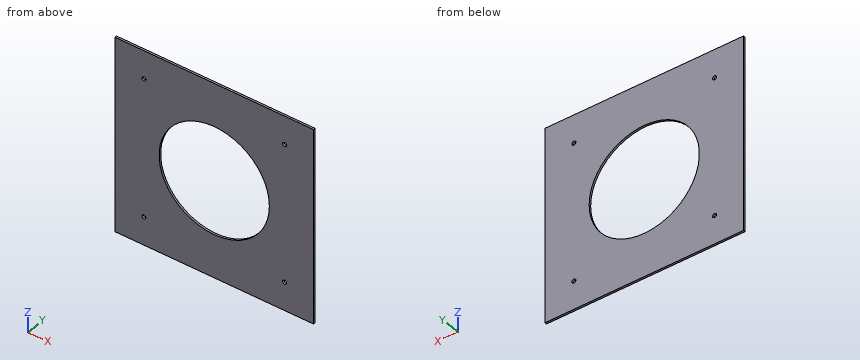
```python
from build123d import *

# Parameters (mm, degrees)
SKETCH1_W           = 98.782817332
SKETCH1_H           = 98.782817332
BOSS_EXTRUDE1_DEPTH = 1.000000032
SKETCH3_R           = 0.999998
CUT_EXTRUDE2_DEPTH  = 2.000000032
SKETCH8_R           = 27.432
CUT_EXTRUDE9_DEPTH  = 2.000000032


with BuildPart() as part:
    # Sketch1 → Boss-Extrude1 (new body)
    with BuildSketch(Plane(origin=(0, 0, 0), x_dir=(1, 0, 0), z_dir=(0, 1, 0))):
        Rectangle(SKETCH1_W, SKETCH1_H)
    extrude(amount=BOSS_EXTRUDE1_DEPTH)

    # Sketch3 → Cut-Extrude2 (cut, through all)
    with BuildSketch(Plane(origin=(0, 0, 0), x_dir=(1, 0, 0), z_dir=(0, 1, 0))):
        with Locations((35.001787507, 35.001787507)):
            Circle(SKETCH3_R)
        with Locations((35.001787507, -35.001787507)):
            Circle(SKETCH3_R)
        with Locations((-35.001787507, -35.001787507)):
            Circle(SKETCH3_R)
        with Locations((-35.001787507, 35.001787507)):
            Circle(SKETCH3_R)
    extrude(amount=CUT_EXTRUDE2_DEPTH, mode=Mode.SUBTRACT)

    # Sketch8 → Cut-Extrude9 (cut, through all)
    with BuildSketch(Plane(origin=(0, 0, 0), x_dir=(1, 0, 0), z_dir=(0, 1, 0))):
        Circle(SKETCH8_R)
    extrude(amount=CUT_EXTRUDE9_DEPTH, mode=Mode.SUBTRACT)


solid = part.part
```
Design review of the part built by this model. Coordinates are the model's own, in mm. Coordinates: 2 decimals unless noted, no trailing zeros. Write each loop counter-clockwise with the first axis right and the second up, starting at its lowest first coordinate (ties: lowest second). Pieces come first, ordered by that corner, then holes.
1) Add section C-C (y = 0.75). Write out the cut boundary in (x, z), plus the area to 3 significant figures.
2) Add section B-B (z = 0). Write out the cut boundary in (x, y), plus the area to 3 significant figures.
3) To check wall thickness, follow L1, parallel to Z at x = 0, y = 0.3; L2, parallel to X at y = 0.25, z = -20; L3, parallel to Z at x = 23, y = 0.5. State the ranges of each line that lie inside material, in increasing order.
4) Insertion check: pin 1 (1.6 mm diameter, centred on x = 35, z = 35, fed in from -Y). The pin has a flat end and moves straight along its axis. Give the tip position at first contact, or say it passes through.
5) Add section A-A (x = 0). Write out the cut boundary in (y, z), plus the area to 3 significant figures.
Check result:
1. outline: (-49.39, -49.39) - (49.39, -49.39) - (49.39, 49.39) - (-49.39, 49.39) - close; hole circle Ø2 at (-35, -35); hole circle Ø2 at (-35, 35); hole circle Ø54.86 at (0, 0); hole circle Ø2 at (35, -35); hole circle Ø2 at (35, 35)
1. area: 7,380 mm2
2. outline: (-49.39, 0) - (-27.43, 0) - (-27.43, 1) - (-49.39, 1) - close; (27.43, 0) - (49.39, 0) - (49.39, 1) - (27.43, 1) - close
2. area: 43.9 mm2
3. L1: z = -49.39 to -27.43, 27.43 to 49.39
3. L2: x = -49.39 to -18.78, 18.78 to 49.39
3. L3: z = -49.39 to -14.95, 14.95 to 49.39
4. pin 1: passes through
5. outline: (0, -49.39) - (1, -49.39) - (1, -27.43) - (0, -27.43) - close; (0, 27.43) - (1, 27.43) - (1, 49.39) - (0, 49.39) - close
5. area: 43.9 mm2
